```python
from build123d import *

# Parameters (mm, degrees)
SKETCH_1_W          = 42
SKETCH_1_H          = 42
SKETCH_1_R          = 11.1
EXTRUDE_1_DEPTH     = 5
SKETCH_2_R          = 1.6
CUT_EXTRUDE_1_DEPTH = 60.607046563
SKETCH_4_W          = 20
SKETCH_4_H          = 9.874323587
EXTRUDE_2_DEPTH     = 20
SKETCH_5_R          = 1.6
CUT_EXTRUDE_2_DEPTH = 20
SKETCH_6_R          = 3
CUT_EXTRUDE_3_DEPTH = 3
EXTRUDE_3_DEPTH     = 9.874324


with BuildPart() as part:
    # 草图1 → 凸台-拉伸1 (new body)
    with BuildSketch(Plane.XY):
        with Locations((21, 21)):
            Rectangle(SKETCH_1_W, SKETCH_1_H)
        with Locations((21, 21)):
            Circle(SKETCH_1_R, mode=Mode.SUBTRACT)
    extrude(amount=EXTRUDE_1_DEPTH)

    # 草图2 → 切除-拉伸1 (cut, through all)
    with BuildSketch(Plane.XY.offset(5)):
        with Locations(Location((36.5, 36.5, 0), (0, 0, 180))):
            Circle(SKETCH_2_R)
        with Locations((5.5, 36.5)):
            Circle(SKETCH_2_R)
        with Locations((36.5, 5.5)):
            Circle(SKETCH_2_R)
        with Locations(Location((5.5, 5.5, 0), (0, 0, 180))):
            Circle(SKETCH_2_R)
    extrude(amount=-CUT_EXTRUDE_1_DEPTH, mode=Mode.SUBTRACT)

    # 草图4 → 凸台-拉伸2 (add)
    with BuildSketch(Plane.XY.offset(5)):
        with Locations((17, 37.062838207)):
            Rectangle(SKETCH_4_W, SKETCH_4_H)
    extrude(amount=EXTRUDE_2_DEPTH)

    # 草图5 → 切除-拉伸2 (cut)
    with BuildSketch(Plane.XZ.offset(-32.125676413)):
        with Locations(Location((17, 21.228996284, 0), (0, 0, 270))):
            Circle(SKETCH_5_R)
        with Locations(Location((17, 9.241211578, 0), (0, 0, 270))):
            Circle(SKETCH_5_R)
    extrude(amount=-CUT_EXTRUDE_2_DEPTH, mode=Mode.SUBTRACT)

    # 草图6 → 切除-拉伸3 (cut)
    with BuildSketch(Plane.XZ.offset(-32.125676413)):
        with Locations(Location((17, 21.228996284, 0), (0, 0, 270))):
            Circle(SKETCH_6_R)
        with Locations(Location((17, 9.241211578, 0), (0, 0, 270))):
            Circle(SKETCH_6_R)
    extrude(amount=-CUT_EXTRUDE_3_DEPTH, mode=Mode.SUBTRACT)

    # 草图7 → 凸台-拉伸3 (add)
    with BuildSketch(Plane.XZ.offset(-32.125676413)):
        Polygon((27, 5), (33.066312707, 5), (27, 25), align=None)
    extrude(amount=-EXTRUDE_3_DEPTH)


solid = part.part
```
The listing builds one solid part. Answer for the finished solid, in the listing's coordinates (mm). A direction names the side the tool comes from. Round coordinates to 2 decimals unless told otherwise and drop trailing zeros. Loops run counter-clockwise (first coordinate to the right, second up) from the corner with the lowest first, then second, coordinate; pieces in that order, holes last.
Q1. Section C-C, the plane x = 5.5 is taken. Determine the outline of the cut face in (y, z), then the cut area to 3 significant figures.
Q2. Which of the six approach directions +Z, -Z, +X, -X, +Y, -Y give full straight-line access (tool end or side, diameter ignored) to faces 1 (the face through (7, 37, 15)), 2 (the face through (15.175, 33.605, 23.61)), 3 (the face through (20, 32.126, 15))?
Q3. For a pull along Y with two mould halves and no side action, classify faces 4 (the face through (3.974, 5.019, 2.535)), 5 (the face through (18.586, 38.515, 9.449)), 6 (the face through (15.7, 35.126, 19.9)), 7 (the face through (31.254, 16.749, 2.465)) as released by +Y, released by -Y, zero draft, split by the parting line, or undercut.
Q4. Section B-B, the plane y = 36.5 is taken. Determine the outline of the cut face in (x, z), then the cut area to 3 significant figures.
Q5. Find the intervals of material crossed by line 1 (Y direction, x = 21, z = 3.65); line 2 (Z direction, x = 39.5, y = 19); line 3 (Y direction, x = 6, z = 1.25), in increasing order.
Q6. Given pin 1 Ø6 at (y, z) = (26, 8.5) entering from +X; pin 2 Ø3 at (x, z) = (17.5, 10.5) entering from -Y; pin 3 Ø21 at (x, y) = (13.5, 19.5) entering from +Z; pin 4 Ø12 at (x, z) = (34.5, 16.5) entering from -Y, each flat-ended and moving along its own axis, determine where each tip first touches the part or whether it passes through.
Completed:
1. outline: (0, 0) - (3.9, 0) - (3.9, 5) - (0, 5) - close; (7.1, 0) - (34.9, 0) - (34.9, 5) - (7.1, 5) - close; (38.1, 0) - (42, 0) - (42, 5) - (38.1, 5) - close
1. area: 178 mm2
2. face 1: +Z, -X, +Y, -Y
2. face 2: -Y
2. face 3: +Z, +X, -X, -Y
3. face 4: undercut
3. face 5: zero draft
3. face 6: released by -Y
3. face 7: undercut
4. outline: (0, 0) - (3.9, 0) - (3.9, 5) - (0, 5) - close; (7, 5) - (7.1, 5) - (7.1, 0) - (34.9, 0) - (34.9, 5) - (33.07, 5) - (27, 25) - (7, 25) - close; (38.1, 0) - (42, 0) - (42, 5) - (38.1, 5) - close; hole circle Ø3.2 at (17, 9.24); hole circle Ø3.2 at (17, 21.23)
4. area: 623 mm2
5. line 1: y = 0 to 9.9, 32.1 to 42
5. line 2: z = 0 to 5
5. line 3: y = 0 to 3.98, 7.02 to 34.98, 38.02 to 42
6. pin 1: passes through
6. pin 2: stops at y = 35.13
6. pin 3: stops at z = 5
6. pin 4: stops at y = 32.13
